from build123d import *

# Parameters (mm, degrees)
CONE009_ANGLE           = 30
CONE007_ANGLE           = 30
CONE008_ANGLE           = 10
CONE008_PLACEMENT_ANGLE = 9.000003


with BuildPart() as obj1:
    # Cone009 → Cone009 (revolve)
    with BuildSketch(Plane(origin=(0, 0, 12), x_dir=(1, 0, 0), z_dir=(0, -1, 0))):
        Polygon((0, 0), (40, 0), (47, 40), (0, 40), align=None)
    revolve(axis=Axis((0, 0, 12), (0, 0, 1)), revolution_arc=CONE009_ANGLE)


with BuildPart() as obj2:
    # Cone007 → Cone007 (revolve)
    with BuildSketch(Plane(origin=(0, 0, 14), x_dir=(1, 0, 0), z_dir=(0, -1, 0))):
        Polygon((0, 0), (42, 0), (50, 38), (0, 38), align=None)
    revolve(axis=Axis((0, 0, 14), (0, 0, 1)), revolution_arc=CONE007_ANGLE)


with BuildPart() as obj3:
    # Cone008 → Cone008 (revolve)
    with BuildSketch(Plane.XZ):
        Polygon((0, 0), (45.5, 0), (51.5, 40), (0, 40), align=None)
    revolve(axis=Axis((0, 0, 0), (0, 0, 1)), revolution_arc=CONE008_ANGLE)


with BuildPart() as obj3_1:
    # Cone008 placement: moved
    add(obj3.part.moved(Location((0, 0, 12))).rotate(Axis((0, 0, 12), (0, 0, 1)), CONE008_PLACEMENT_ANGLE))

    # Cut006: cut obj2
    add(obj2.part, mode=Mode.SUBTRACT)

    # Cut007: cut obj1
    add(obj1.part, mode=Mode.SUBTRACT)


solid = obj3_1.part
For this review, take the finished solid that the model builds, in its own axes (mm). A direction names the side the tool comes from. Give positions to 0.01 mm unless a question says otherwise; leave off trailing zeros. Order: outer loops, then holes, each group sorted by start corner. A loop starts at its lowest first (then second) coordinate and runs counter-clockwise, first axis right, second up. Notation, with made-up numbers: (42.5, -31.75) - (92.5, -31.75) arc R34 ccw to (92.5, 3.25) - close; hole circle Ø3 at (47, 41.5). An arc over 180 degrees is marked (long way). Answer as a JSON object with one key per item and string values. Group by question number.
Item 1: Clearance check with flat-ended pins moving along their axes: pin 1 Ø5 at (x, z) = (42, 22.5) entering from +Y; pin 2 Ø2 at (y, z) = (9, 43.5) entering from -X; pin 3 Ø5 at (x, z) = (43, 19.5) entering from -Y; pin 4 Ø3 at (x, y) = (47, 13.5) entering from +Z. State where each tip first meets the part, or that it passes through.
Item 2: Take a section at B-B on z = 32.5. Give the boundary of the cut face in (x, y) (3 decimals), and give its area (3 significant figures).
Item 3: Machinability: for faces 1 (the flat face through (40, 10, 14)), 2 (the flat face through (41, 11, 12)), which of the approach directions +Z, -Z, +X, -X, +Y, -Y give a long, thin tool a straight path to every point of the face, cutting with its end or side? Answer none if there is none.
Item 4: Take a section at A-A on z = 24.5. Give the boundary of the cut face in (x, y) (3 decimals), and give its area (3 significant figures).
Item 5: Wall thickness on line 1 along Z through (x, y) = (40, 11.5); line 2 along X through (y, z) = (8, 29.5); line 3 along X through (y, z) = (9.75, 27): over which ranges is each line inside the solid? List them lowest first.
Reported:
{
 "1": {"pin 1": "y = 15.32", "pin 2": "x = 47.07", "pin 3": "y = 6.67", "pin 4": "z = 52"},
 "2": {"outline": "(43.394, 14.942) arc R45.895 cw to (45.33, 7.18) - (47.977, 7.599) arc R48.575 ccw to (45.929, 15.814) - close", "area": "22.1 mm^2"},
 "3": {"face 1": "+Z, -X, -Y", "face 2": "-Z, +X, -X, +Y, -Y"},
 "4": {"outline": "(41.802, 14.394) arc R44.211 cw to (43.666, 6.916) - (46.792, 7.411) arc R47.375 ccw to (44.794, 15.424) - close", "area": "25.3 mm^2"},
 "5": {"line 1": "12 to 14", "line 2": "44.55 to 47.46", "line 3": "43.66 to 46.74"}
}
